Build history of the part. All positions in model axes, mm. A direction names the side the tool comes from. Give positions to 0.01 mm unless a question says otherwise; leave off trailing zeros. Loops run counter-clockwise (first coordinate to the right, second up) from the corner with the lowest first, then second, coordinate; pieces in that order, holes last.
1) Band-saw the part on A-A on z = 2.75. List the corners of the cut face in (x, y).
2) 3-axis set-ups, long thin cutter, end or side, ignore diameter. For faces 1 (the flat face through (2.444, 4.362, 1.479)), 2 (the flat face through (0, 0, 2)): which of +Z, -Z, +X, -X, +Y, -Y reach the whole face in a straight line?
3) Band-saw the part on D-D on x = 4.75. List the corners of the cut face in (y, z), then the cut area to 3 significant figures.
4) Band-saw the part on C-C on z = 1. List the corners of the cut face in (x, y), then the cut area to 3 significant figures.
5) Flat gauge pins, fed straight in: P1, Ø6, axis at x = -1, y = 1.5, coming from the +Z side; P2, Ø5, axis at y = -2.5, z = 5, coming from the -X side; P3, Ø4, axis at y = 0.5, z = 6, coming from the -X side; P4, Ø5, axis at x = -2, z = 6, coming from the -Y side. Where does each tip first touch, or does it go through?
6) Band-saw the part on B-B on y = 0.75. List the corners of the cut face in (x, z), then the cut area to 3 significant figures.
7) Wall check: line 1 (Y direction, x = 0, z = 7); line 2 (X direction, y = -1, z = 6); line 3 (Z direction, x = 1.5, y = -1.25). Give the ranges that are in metal, low to high.
Autodesk Inventor part; units mm, degrees
ref_plane "YZ Plane" through (0, 0, 0) normal (1, 0, 0) x (0, 1, 0)
ref_plane "XZ Plane" through (0, 0, 0) normal (0, 1, 0) x (-1, 0, 0)
ref_plane "XY Plane" through (0, 0, 0) normal (0, 0, 1) x (1, 0, 0)
sketch "Boceto1" plane through (0, 0, 0) normal (0, 0, 1) x (1, 0, 0)
  line L0 (5.0141, -2.8621) -> (0.0284, -5.7734)
  line L1 (0.0284, -5.7734) -> (-4.9858, -2.9113)
  line L2 (-4.9858, -2.9113) -> (-5.0141, 2.8621)
  line L3 (-5.0141, 2.8621) -> (-0.0284, 5.7734)
  line L4 (-0.0284, 5.7734) -> (4.9858, 2.9113)
  line L5 (4.9858, 2.9113) -> (5.0141, -2.8621)
  point P0 (0, 0)
  point P1 (0, 0)
  dimension "d0" = 10
extrude "Extrusión1" add sketch "Boceto1" along normal blind 3
sketch "Boceto2" plane through (0, 0, 3) normal (0, 0, 1) x (1, 0, 0)
  circle A0 centre (0, 0) radius 4
  circle A1 centre (0, 0) radius 2.5
  dimension "d3" = 8
  dimension "d4" = 5
extrude "Extrusión2" add sketch "Boceto2" along normal blind 6 contours A0 | A1
sketch "Boceto3" plane through (0, 0, 9) normal (0, 0, 1) x (1, 0, 0)
  point P0 (0, 0)
  point P1 (0, 0)
hole "Agujero1" at (0, 0, 9) direction (0, 0, -1) diameter 5 depth 7
thread "Rosca1"
properties part number "Hudson 1-57"
Findings below:
1. outline: (-5.01, 2.86) - (-4.99, -2.91) - (0.03, -5.77) - (5.01, -2.86) - (4.99, 2.91) - (-0.03, 5.77) - close; hole circle Ø5 at (0, 0)
2. face 1: +Z, -Z, +X, +Y
2. face 2: +Z
3. outline: (-3.02, 0) - (3.05, 0) - (3.05, 3) - (-3.02, 3) - close
3. area: 18.2 mm2
4. outline: (-5.01, 2.86) - (-4.99, -2.91) - (0.03, -5.77) - (5.01, -2.86) - (4.99, 2.91) - (-0.03, 5.77) - close
4. area: 86.6 mm2
5. P1: stops at z = 9
5. P2: stops at x = -5
5. P3: stops at x = -4
5. P4: stops at y = -4
6. outline: (-5, 0) - (5, 0) - (5, 3) - (3.93, 3) - (3.93, 9) - (2.38, 9) - (2.38, 2) - (-2.38, 2) - (-2.38, 9) - (-3.93, 9) - (-3.93, 3) - (-5, 3) - close
6. area: 43.8 mm2
7. line 1: y = -4 to -2.5, 2.5 to 4
7. line 2: x = -3.87 to -2.29, 2.29 to 3.87
7. line 3: z = 0 to 2
